```python
from build123d import *

# Parameters (mm, degrees)
F0_W     = 3
F0_H     = 8.4
F1_DEPTH = 24


with BuildPart() as f1:
    # F0 (on Top) → F1 (new body)
    with BuildSketch(Plane.XY):
        with BuildLine():
            Line((0, 11.3), (0, 0))
            ThreePointArc((0, 0), (5, -25.136427), (10, 0))
            Line((10, 0), (10, 31))
            ThreePointArc((10, 31), (5, 56.136427), (0, 31))
            Line((0, 31), (0, 19.7))
            Line((0, 19.7), (0, 11.3))
        make_face()
        with BuildLine():
            ThreePointArc((2, 32.419858), (5, 54.136427), (8, 32.419858))
            Line((8, 32.419858), (8, -1.419858))
            ThreePointArc((8, -1.419858), (5, -23.136427), (2, -1.419858))
            Line((2, -1.419858), (2, 32.419858))
        make_face(mode=Mode.SUBTRACT)
        with Locations((-1.5, 15.5)):
            Rectangle(F0_W, F0_H)
    extrude(amount=F1_DEPTH)


solid = f1.part
```
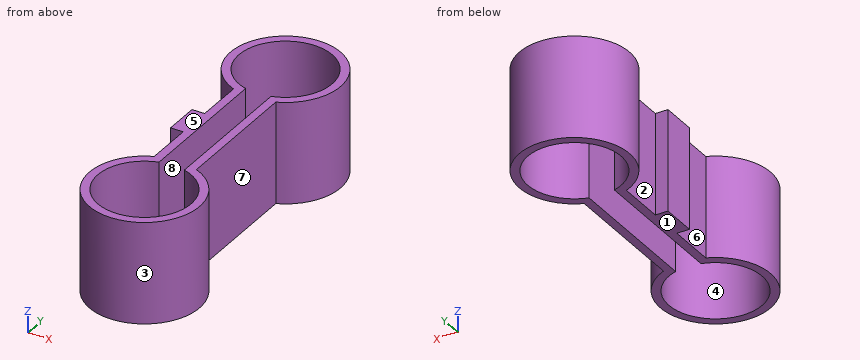
Could you check a few things on this model? Use its own coordinates, in mm. Face numbers are marked on the shaded views. A direction names the side the tool comes from. Give positions to 0.01 mm unless a question says otherwise; leave off trailing zeros. Loops run counter-clockwise (first coordinate to the right, second up) from the corner with the lowest first, then second, coordinate; pieces in that order, holes last. Notation, with made-up numbers: (-33.5, 58) - (-3.5, 58) arc R17 ccw to (-3.5, 84) - close; hole circle Ø2 at (29.25, 24). An arc over 180 degrees is marked (long way). Use one line per item in the form item = value.
1. I want a section at A-A (y = 2). Please give me the cut outline in (x, z).
Response values:
outline = (0, 0) - (2, 0) - (2, 24) - (0, 24) - close; (8, 0) - (10, 0) - (10, 24) - (8, 24) - close
2. I need wall thicknesses on probe 1 along X at (y, z) = (11, 11.75); probe 2 along Y at (x, z) = (11, 17.5); probe 3 along X at (y, z) = (43.5, 17.75). Which ranges of each line are inside material? Lowest first, please.
Response values:
probe_1 = 0 to 2, 8 to 10
probe_2 = -23.68 to -21.37, -2.77 to -0.46, 31.46 to 33.77, 52.37 to 54.68
probe_3 = -8.06 to -6.06, 16.06 to 18.06
3. I want a section at C-C (z = 7.25). Please give me the cut outline in (x, y), and give its area (3 significant figures).
Response values:
outline = (-3, 11.3) - (0, 11.3) - (0, 0) arc R13.07 ccw (long way) to (10, 0) - (10, 31) arc R13.07 ccw (long way) to (0, 31) - (0, 19.7) - (-3, 19.7) - close; hole (2, -1.42) arc R11.07 ccw (long way) to (8, -1.42) - (8, 32.42) arc R11.07 ccw (long way) to (2, 32.42) - close
area = 425 mm²
4. Thinking about a two-plate mould opening in X: for the marked faces 1, 2, 3 and 4, which applies, released by +X, released by -X, zero draft, split by the parting line, or undercut?
Response values:
face_1 = zero draft
face_2 = released by -X
face_3 = split by the parting line
face_4 = undercut
5. I want a section at D-D (x = 12.5). Please give me the cut outline in (y, z), and give its area (3 significant figures).
Response values:
outline = (-22.77, 0) - (-20.21, 0) - (-20.21, 24) - (-22.77, 24) - close; (-3.93, 0) - (-1.37, 0) - (-1.37, 24) - (-3.93, 24) - close; (32.37, 0) - (34.93, 0) - (34.93, 24) - (32.37, 24) - close; (51.21, 0) - (53.77, 0) - (53.77, 24) - (51.21, 24) - close
area = 246 mm²
6. I'm going to push flat-ended pins straight in: pin 1 Ø3.5 at (y, z) = (23.5, 17) entering from -X; pin 2 Ø10 at (y, z) = (1.5, 20) entering from +X; pin 3 Ø9 at (y, z) = (14, 10) entering from -X; pin 4 Ø13.5 at (x, y) = (5, -12.07) entering from -Z. Where does each tip first touch, or does it pass through?
Response values:
pin_1 = 0
pin_2 = 14.86
pin_3 = -3
pin_4 = through
7. On a 3-axis mill with a long thin cutter (end or side, diameter ignored), from which of +Z, -Z, +X, -X, +Y, -Y can I reach the whole of each face in a straight line? I mean the marked faces 5, 6, 7 and 8. Say none if no direction works.
Response values:
face_5 = +Z, +X, -X, +Y, -Y
face_6 = +Z, -Z, -X
face_7 = +Z, -Z, +X
face_8 = +Z, -Z
8. I want a section at B-B (x = 5). Please give me the cut outline in (y, z), and give its area (3 significant figures).
Response values:
outline = (-25.14, 0) - (-23.14, 0) - (-23.14, 24) - (-25.14, 24) - close; (54.14, 0) - (56.14, 0) - (56.14, 24) - (54.14, 24) - close
area = 96.0 mm²
